Can you work these out from the model? Positions are in its coordinate system, mm. Face numbers are marked on the shaded views. A direction names the side the tool comes from. Coordinates: 2 decimals unless noted, no trailing zeros. Order: outer loops, then holes, each group sorted by start corner. A loop starts at its lowest first (then second) coordinate and runs counter-clockwise, first axis right, second up. Notation, with made-up numbers: (29, 9.25) -> (61, 9.25) arc R21 ccw to (61, 15.25) -> close; hole circle Ø11 at (18.5, -7.75). An arc over 180 degrees is marked (long way). Answer in a Markdown table with one row per item.
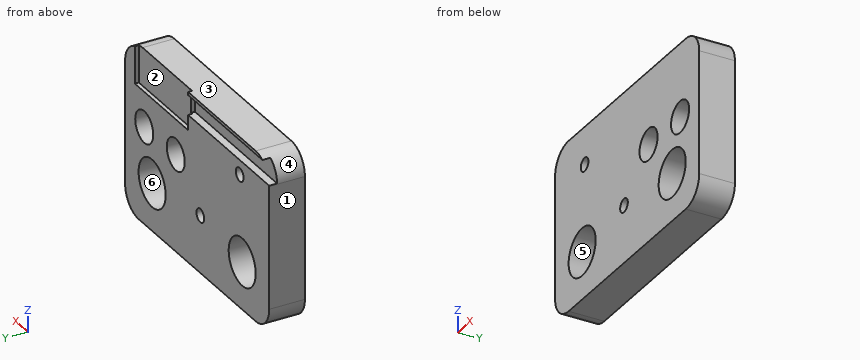
```python
from build123d import *

# Parameters (mm, degrees)
SKETCH034_R     = 6
SKETCH034_R_2   = 4
SKETCH034_R_3   = 1.7
PAD010_DEPTH    = 9
SKETCH035_W     = 23.67814
SKETCH035_H     = 16.3581
POCKET022_DEPTH = 1
SKETCH036_W     = 37.866951
SKETCH036_H     = 5
POCKET023_DEPTH = 2


with BuildPart() as part:
    # Sketch034 → Pad010 (new body)
    with BuildSketch(Plane.XZ):
        with BuildLine():
            Line((38.838751, 1.547306), (-13.161249, 1.547306))
            ThreePointArc((-13.161249, 1.547306), (-17.40389, -0.210054), (-19.161249, -4.452694))
            Line((-19.161249, -4.452694), (-19.161249, -35.452694))
            ThreePointArc((-19.161249, -35.452694), (-17.40389, -39.695335), (-13.161249, -41.452694))
            Line((-13.161249, -41.452694), (38.838751, -41.452694))
            ThreePointArc((38.838751, -41.452694), (43.081392, -39.695335), (44.838751, -35.452694))
            Line((44.838751, -35.452694), (44.838751, -4.452694))
            ThreePointArc((44.838751, -4.452694), (43.081392, -0.210054), (38.838751, 1.547306))
        make_face()
        with Locations((32.838751, -29.452694)):
            Circle(SKETCH034_R, mode=Mode.SUBTRACT)
        with Locations((-7.161249, -29.452694)):
            Circle(SKETCH034_R, mode=Mode.SUBTRACT)
        with Locations((22.338751, -16.952694)):
            Circle(SKETCH034_R_2, mode=Mode.SUBTRACT)
        with Locations((36.338751, -16.952694)):
            Circle(SKETCH034_R_2, mode=Mode.SUBTRACT)
        with Locations((11.438751, -26.952694)):
            Circle(SKETCH034_R_3, mode=Mode.SUBTRACT)
        with Locations((-6.061249, -7.952694)):
            Circle(SKETCH034_R_3, mode=Mode.SUBTRACT)
    extrude(amount=PAD010_DEPTH)

    # Sketch035 (on Face15 of Pad010) → Pocket022 (cut)
    with BuildSketch(Plane(origin=(0, 0, 0), x_dir=(1, 0, 0), z_dir=(0, 1, 0))):
        with Locations((28.687662, -0.089719)):
            Rectangle(SKETCH035_W, SKETCH035_H)
    extrude(amount=-POCKET022_DEPTH, mode=Mode.SUBTRACT)

    # Sketch036 (on Face4 of Pocket022) → Pocket023 (cut)
    with BuildSketch(Plane(origin=(0, 0, 0), x_dir=(1, 0, 0), z_dir=(0, 1, 0))):
        with Locations((-1.591031, 1.759919)):
            Rectangle(SKETCH036_W, SKETCH036_H)
    extrude(amount=-POCKET023_DEPTH, mode=Mode.SUBTRACT)


with BuildPart() as part_1:
    # Body004 placement: moved
    add(part.part.moved(Location((-2.5, -18, 1.5))))


solid = part_1.part
```
(1) Will these pins go through, and if not, where does the flat tip stop? pin 1 Ø1.1 at (y, z) = (-19.5, -1.5) entering from -X; pin 2 Ø1.1 at (y, z) = (-18.5, -1) entering from -X; pin 3 Ø0.8 at (x, y) = (30.5, -18.5) entering from +Z.
Response values:
| item | result |
|---|---|
| pin 1 | x = -21.54 |
| pin 2 | x = 14.84 |
| pin 3 | z = -6.59 |
(2) Suppose I cut it at A-A (x = -7.5). Please give me the cut outline in (y, z).
Response values:
| item | result |
|---|---|
| outline | (-27, -39.95) -> (-18, -39.95) -> (-18, -33.55) -> (-27, -33.55) -> close; (-27, -22.36) -> (-18, -22.36) -> (-18, -7.78) -> (-27, -7.78) -> close; (-27, -5.12) -> (-18, -5.12) -> (-18, -2.76) -> (-20, -2.76) -> (-20, 2.24) -> (-18, 2.24) -> (-18, 3.05) -> (-27, 3.05) -> close |
(3) Suppose I cut it at C-C (y = -22). Please give me the cut outline in (x, z), and give its area (3 significant figures).
Response values:
| item | result |
|---|---|
| outline | (-21.66, -33.95) arc R6 ccw to (-15.66, -39.95) -> (36.34, -39.95) arc R6 ccw to (42.34, -33.95) -> (42.34, -2.95) arc R6 ccw to (36.34, 3.05) -> (-15.66, 3.05) arc R6 ccw to (-21.66, -2.95) -> close; hole circle Ø12 at (-9.66, -27.95); hole circle Ø3.4 at (-8.56, -6.45); hole circle Ø3.4 at (8.94, -25.45); hole circle Ø8 at (19.84, -15.45); hole circle Ø12 at (30.34, -27.95); hole circle Ø8 at (33.84, -15.45) |
| area | 2,380 mm2 |
(4) We'd pull the mould along X, two halves only. Please class the marked faces 3, 4, 5 and 6: +X half, -X half, draft (parallel to the pull), parting line (faces both ways), or undercut.
Response values:
| item | result |
|---|---|
| face 3 | draft |
| face 4 | -X half |
| face 5 | undercut |
| face 6 | undercut |
(5) On a 3-axis mill with a long thin cutter (end or side, diameter ignored), from which of +Z, -Z, +X, -X, +Y, -Y can I reach the whole of each face in a straight line? I mean the marked faces 1 and 2. Say none if no direction works.
Response values:
| item | result |
|---|---|
| face 1 | +Z, -Z, -X, +Y, -Y |
| face 2 | +Z, +Y |
(6) Suppose I cut it at D-D (z = -29.5). Please give me the cut outline in (x, y), and give its area (3 significant figures).
Response values:
| item | result |
|---|---|
| outline | (-21.66, -27) -> (-15.46, -27) -> (-15.46, -18) -> (-21.66, -18) -> close; (-3.86, -27) -> (24.54, -27) -> (24.54, -18) -> (-3.86, -18) -> close; (36.14, -27) -> (42.34, -27) -> (42.34, -18) -> (36.14, -18) -> close |
| area | 367 mm2 |
(7) Suppose I cut it at B-B (x = 18.5). Please give me the cut outline in (y, z), and give its area (3 significant figures).
Response values:
| item | result |
|---|---|
| outline | (-27, -39.95) -> (-18, -39.95) -> (-18, -19.22) -> (-27, -19.22) -> close; (-27, -11.68) -> (-18, -11.68) -> (-18, -6.59) -> (-19, -6.59) -> (-19, 3.05) -> (-27, 3.05) -> close |
| area | 310 mm2 |
(8) I need wall thicknesses on line 1 (X direction, y = -20.5, z = -16); line 2 (Z direction, x = 34.5, y = -19.75); line 3 (X direction, y = -26, z = -18). Which ranges of each line are inside material? Lowest first, please. Write a range as [from, to].
Response values:
| item | result |
|---|---|
| line 1 | [-21.66, 15.88], [23.8, 29.88], [37.8, 42.34] |
| line 2 | [-39.95, -32.28], [-23.63, -19.4], [-11.51, 3.05] |
| line 3 | [-21.66, 16.75], [22.92, 30.75], [36.92, 42.34] |
